from build123d import *

# Parameters (mm, degrees)
SKETCH5_R           = 13.505404748
BOSS_EXTRUDE1_DEPTH = 1.6256
SKETCH6_W           = 19.854
SKETCH6_H           = 13.254
CUT_EXTRUDE1_DEPTH  = 20.168580808
SKETCH7_R           = 0.508
CUT_EXTRUDE2_DEPTH  = 20.168580808
SKETCH9_R           = 0.467957387
SKETCH9_R_2         = 0.471151672
SKETCH9_R_3         = 0.612350227
BOSS_EXTRUDE2_DEPTH = 1.778
SKETCH10_R          = 13.5128
BOSS_EXTRUDE3_DEPTH = 1.6256
SKETCH11_W          = 27.94
SKETCH11_H          = 7.366
BOSS_EXTRUDE4_DEPTH = 1.6256
SKETCH12_R          = 0.381
BOSS_EXTRUDE5_DEPTH = 2.54


with BuildPart() as part:
    # Sketch5 → Boss-Extrude1 (new body)
    with BuildSketch(Plane.XY):
        Circle(SKETCH5_R)
    extrude(amount=BOSS_EXTRUDE1_DEPTH)

    # Sketch6 → Cut-Extrude1 (cut, through all)
    with BuildSketch(Plane.XY.offset(1.6256)):
        Rectangle(SKETCH6_W, SKETCH6_H)
    extrude(amount=-CUT_EXTRUDE1_DEPTH, mode=Mode.SUBTRACT)

    # Sketch7 → Cut-Extrude2 (cut, through all)
    with BuildSketch(Plane.XY.offset(1.6256)):
        with Locations((-9.927, 6.119)):
            Circle(SKETCH7_R)
        with Locations((-9.927, -6.119)):
            Circle(SKETCH7_R)
        with Locations((9.927, -6.119)):
            Circle(SKETCH7_R)
        with Locations((9.927, 6.119)):
            Circle(SKETCH7_R)
    extrude(amount=-CUT_EXTRUDE2_DEPTH, mode=Mode.SUBTRACT)

    # Sketch9 → Boss-Extrude2 (add)
    with BuildSketch(Plane(origin=(0, 0, 0), x_dir=(-1, 0, 0), z_dir=(0, 0, -1))):
        with Locations(Location((-6.791513401, 10.433736314, 0), (0, 0, 180))):
            Circle(SKETCH9_R)
        with Locations(Location((6.243810708, 10.901693701, 0), (0, 0, 180))):
            Circle(SKETCH9_R_2)
        with Locations(Location((5.422256667, -10.76235793, 0), (0, 0, 180))):
            Circle(SKETCH9_R_3)
        with Locations(Location((-6.791513401, -10.150007703, 0), (0, 0, 180))):
            Circle(SKETCH9_R_3)
    extrude(amount=BOSS_EXTRUDE2_DEPTH)

    # Sketch10 → Boss-Extrude3 (add)
    with BuildSketch(Plane(origin=(0, 0, -1.778), x_dir=(-1, 0, 0), z_dir=(0, 0, -1))):
        Circle(SKETCH10_R)
    extrude(amount=BOSS_EXTRUDE3_DEPTH)

    # Sketch11 → Boss-Extrude4 (add)
    with BuildSketch(Plane(origin=(0, 0, -3.4036), x_dir=(-1, 0, 0), z_dir=(0, 0, -1))):
        Rectangle(SKETCH11_W, SKETCH11_H)
    extrude(amount=-BOSS_EXTRUDE4_DEPTH)

    # Sketch12 → Boss-Extrude5 (add)
    with BuildSketch(Plane(origin=(0, 0, -3.4036), x_dir=(-1, 0, 0), z_dir=(0, 0, -1))):
        with Locations((-11.43, 0)):
            Circle(SKETCH12_R)
        with Locations(Location((11.43, 0, 0), (0, 0, 180))):
            Circle(SKETCH12_R)
    extrude(amount=BOSS_EXTRUDE5_DEPTH)


solid = part.part
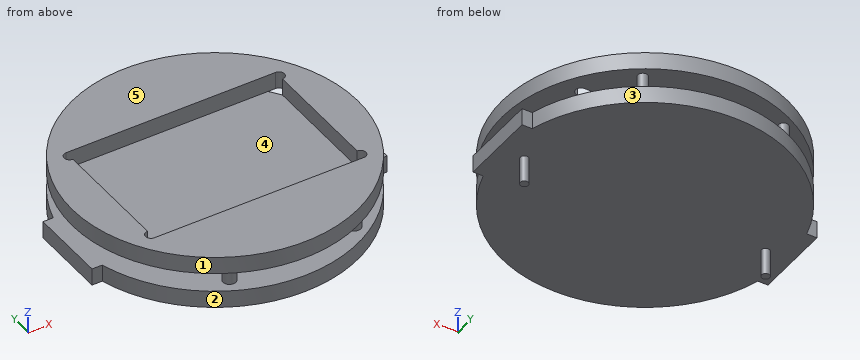
Design review of the part built by this model. Coordinates are the model's own, in mm. Face numbers are marked on the shaded views. A direction names the side the tool comes from. Round coordinates to 2 decimals unless told otherwise and drop trailing zeros. Write each loop counter-clockwise with the first axis right and the second up, starting at its lowest first coordinate (ties: lowest second). Pieces come first, ordered by that corner, then holes.
Item 1: Consider section B-B on y = 0. Give the boundary of the cut face in (x, z), and give its area (3 significant figures).
Item 2: For the marked faces 1 and 2, list the 3-axis set-ups (+Z, -Z, +X, -X, +Y, -Y) from which the entire face can be reached by the end or side of a thin tool; tool diameter is ignored.
Item 3: Wall thickness on L1, parallel to Z at x = 2.5, y = -12; L2, parallel to Z at x = -0.25, y = 0; L3, parallel to Y at x = -3.5, z = 1: over which ranges is each line inside the solid? List them lowest first.
Item 4: Draft analysis for pull direction Z (two halves, no side actions). For the marked faces 3, 4 and 5, state which applies: released by +Z, released by -Z, zero draft, split by the parting line, or undercut.
Item 5: For pin 1 Ø1 at (x, z) = (0, -1.5) entering from +Y; pin 2 Ø0.8 at (x, z) = (-13.5, -3) entering from +Y; pin 3 Ø1.3 at (x, z) = (-4.5, 1) entering from +Y (3 decimals); pin 4 Ø8 at (x, y) = (2.5, -4) entering from -Z, all flat-tipped, find the tip position at first contact; note any pin that passes through.
Item 6: Consider section A-A on x = 0. Give the boundary of the cut face in (y, z), and give its area (3 significant figures).
Item 7: Consider section C-C on z = 1. Give the boundary of the cut face in (x, y).
Item 8: Consider section D-D on x = 12.25. Give the boundary of the cut face in (y, z).
Check values:
1. outline: (-13.97, -3.4) - (-11.81, -3.4) - (-11.81, -5.94) - (-11.05, -5.94) - (-11.05, -3.4) - (11.05, -3.4) - (11.05, -5.94) - (11.81, -5.94) - (11.81, -3.4) - (13.97, -3.4) - (13.97, -1.78) - (-13.97, -1.78) - close; (-13.51, 0) - (-9.93, 0) - (-9.93, 1.63) - (-13.51, 1.63) - close; (9.93, 0) - (13.51, 0) - (13.51, 1.63) - (9.93, 1.63) - close
1. area: 60.9 mm2
2. face 1: +Z
2. face 2: +Z, -Z, -Y
3. L1: z = -3.4 to -1.78, 0 to 1.63
3. L2: z = -3.4 to -1.78
3. L3: y = -13.04 to -6.63, 6.63 to 13.04
4. face 3: zero draft
4. face 4: undercut
4. face 5: released by +Z
5. pin 1: stops at y = 13.51
5. pin 2: stops at y = 3.68
5. pin 3: stops at y = 12.945
5. pin 4: stops at z = -3.4
6. outline: (-13.51, -3.4) - (13.51, -3.4) - (13.51, -1.78) - (-13.51, -1.78) - close; (-13.51, 0) - (-6.63, 0) - (-6.63, 1.63) - (-13.51, 1.63) - close; (6.63, 0) - (13.51, 0) - (13.51, 1.63) - (6.63, 1.63) - close
6. area: 66.3 mm2
7. outline: circle Ø27.01 at (0, 0); hole (-9.93, -6.63) - (9.93, -6.63) arc R0.51 ccw to (9.93, -5.61) - (9.93, 5.61) arc R0.51 ccw to (9.93, 6.63) - (-9.93, 6.63) arc R0.51 ccw to (-9.93, 5.61) - (-9.93, -5.61) arc R0.51 ccw to start
8. outline: (-5.7, -3.4) - (5.7, -3.4) - (5.7, -1.78) - (-5.7, -1.78) - close; (-5.69, 0) - (5.69, 0) - (5.69, 1.63) - (-5.69, 1.63) - close
